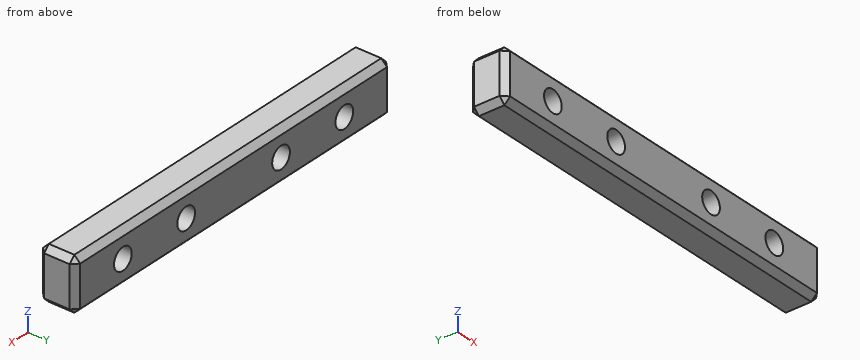
from build123d import *

# Parameters (mm, degrees)
SCHIZZO1_W                   = 100
SCHIZZO1_H                   = 13.6
ESTRUSIONE_ESTRUSIONE1_DEPTH = 9.6
FORO_5_6_5_6_1_D             = 5.6
SMUSSO1_SIZE                 = 1.5


with BuildPart() as part:
    # Schizzo1 → Estrusione-Estrusione1 (new body)
    with BuildSketch(Plane(origin=(0, 4.8, 0), x_dir=(1, 0, 0), z_dir=(0, 1, 0))):
        Rectangle(SCHIZZO1_W, SCHIZZO1_H)
    extrude(amount=-ESTRUSIONE_ESTRUSIONE1_DEPTH)

    # Foro Ø5.6 (5.6)-1 (through all)
    with Locations(Plane(origin=(0, -4.8, 0), x_dir=(-1, 0, 0), z_dir=(0, -1, 0))):
        with Locations((-35, 0), (35, 0), (-15, 0), (15, 0)):
            Hole(FORO_5_6_5_6_1_D / 2)

    # Smusso1
    smusso1_edges = [part.edges().sort_by_distance(p)[0] for p in [
        (0, -4.8, -6.8),
        (-50, -4.8, 0),
        (0, -4.8, 6.8),
        (-50, 4.8, 0),
        (0, 4.8, -6.8),
        (50, 4.8, 0),
        (0, 4.8, 6.8),
        (-50, 0, 6.8),
        (-50, 0, -6.8),
        (50, 0, -6.8),
        (50, 0, 6.8),
        (50, -4.8, 0),
    ]]
    chamfer(smusso1_edges, length=SMUSSO1_SIZE)


solid = part.part
Source: CAD feature listing. Evaluate the final solid. Frame: model axes, mm. Coordinates: 2 decimals unless noted, no trailing zeros. Loops run counter-clockwise (first coordinate to the right, second up) from the corner with the lowest first, then second, coordinate; pieces in that order, holes last. Notation, with made-up numbers: (-28.5, 77) -> (-14.5, 77) arc R18 cw to (-14.5, 96) -> close; hole circle Ø7 at (5.25, -26). An arc over 180 degrees is marked (long way). Answer in a Markdown table with one row per item. Add a question column.
Q1. Ray query, line 1 along X through (y, z) = (-1.5, 0.5) (3 decimals); line 2 along Z through (x, y) = (-35, 1.75); line 3 along X through (y, z) = (3, -2). Return the intervals inside material, ascending.
Q2. Section B-B on x = -15. Return the cut outline in (y, z), and give its area (3 significant figures).
Q3. Section A-A on z = 0. Return the cut outline in (x, y).
Q4. Section C-C on y = -1.25. Return the cut outline in (x, z).
Computed values:
| question | item | result |
|---|---|---|
| 1 | line 1 | x = -50 to -37.755, -32.245 to -17.755, -12.245 to 12.245, 17.755 to 32.245, 37.755 to 50 |
| 1 | line 2 | z = -6.8 to -2.8, 2.8 to 6.8 |
| 1 | line 3 | x = -50 to -36.96, -33.04 to -16.96, -13.04 to 13.04, 16.96 to 33.04, 36.96 to 50 |
| 2 | outline | (-4.8, -5.3) -> (-3.3, -6.8) -> (3.3, -6.8) -> (4.8, -5.3) -> (4.8, -2.8) -> (-4.8, -2.8) -> close; (-4.8, 2.8) -> (4.8, 2.8) -> (4.8, 5.3) -> (3.3, 6.8) -> (-3.3, 6.8) -> (-4.8, 5.3) -> close |
| 2 | area | 72.3 mm^2 |
| 3 | outline | (-50, -3.3) -> (-48.5, -4.8) -> (-37.8, -4.8) -> (-37.8, 4.8) -> (-48.5, 4.8) -> (-50, 3.3) -> close; (-32.2, -4.8) -> (-17.8, -4.8) -> (-17.8, 4.8) -> (-32.2, 4.8) -> close; (-12.2, -4.8) -> (12.2, -4.8) -> (12.2, 4.8) -> (-12.2, 4.8) -> close; (17.8, -4.8) -> (32.2, -4.8) -> (32.2, 4.8) -> (17.8, 4.8) -> close; (37.8, -4.8) -> (48.5, -4.8) -> (50, -3.3) -> (50, 3.3) -> (48.5, 4.8) -> (37.8, 4.8) -> close |
| 4 | outline | (-50, -5.3) -> (-48.5, -6.8) -> (48.5, -6.8) -> (50, -5.3) -> (50, 5.3) -> (48.5, 6.8) -> (-48.5, 6.8) -> (-50, 5.3) -> close; hole circle Ø5.6 at (-35, 0); hole circle Ø5.6 at (-15, 0); hole circle Ø5.6 at (15, 0); hole circle Ø5.6 at (35, 0) |
